Autodesk Inventor part; units mm, degrees
ref_plane "to_screw1_XY" through (15, 4.2426, 4.2426) normal (0, 0.7071, 0.7071) x (1, 0, 0)
ref_plane "to_screw1_YZ" through (15, 4.2426, 4.2426) normal (1, 0, 0) x (0, 0.7071, -0.7071)
ref_plane "to_screw1_ZX" through (15, 4.2426, 4.2426) normal (0, 0.7071, -0.7071) x (0, 0.7071, 0.7071)
sketch "Sketch_1" plane through (0, 0, 0) normal (0, 0, 1) x (1, 0, 0)
  line L0 (24, 0) -> (0, 0)
  line L1 (0, 18) -> (0, 6)
  line L2 (0, 6) -> (24, 6)
  line L3 (24, 6) -> (24, 8)
  line L4 (24, 8) -> (6, 8)
  line L5 (6, 8) -> (6, 18)
  line L6 (6, 18) -> (0, 18)
revolve "Revolution1" add sketch "Sketch_1" angle 360 about axis through (24, 0, 0) along (1, 0, 0)
sketch "Sketch_3" plane through (0, 0, 0) normal (0, -0.7071, 0.7071) x (1, 0, 0)
  line L0 (15, 5.5) -> (15, 8)
  line L1 (15, 8) -> (17, 8)
  line L2 (17, 8) -> (16.621, 7.621)
  line L3 (16.621, 7.621) -> (16.621, 5.5)
  line L4 (16.621, 5.5) -> (15, 5.5)
  line L5 (15, 5.5) -> (15, 8)
revolve "Revolution2" cut sketch "Sketch_3" angle 360 about axis through (15, 3.8891, 3.8891) along (0, -0.7071, -0.7071)
thread "Thread1"
sketch "Sketch_2" plane through (0, 0, 0) normal (0, -0.7071, -0.7071) x (1, 0, 0)
  line L0 (15, 5.5) -> (15, 8)
  line L1 (15, 8) -> (17, 8)
  line L2 (17, 8) -> (16.621, 7.621)
  line L3 (16.621, 7.621) -> (16.621, 5.5)
  line L4 (16.621, 5.5) -> (15, 5.5)
  line L5 (15, 5.5) -> (15, 8)
revolve "Revolution3" cut sketch "Sketch_2" angle 360 about axis through (15, -3.8891, 3.8891) along (0, 0.7071, -0.7071)
thread "Thread2"
sketch "Sketch_4" plane through (0, 0, 0) normal (0, 0, 1) x (1, 0, 0)
  line L0 (6, 13) -> (0, 13)
  line L1 (0, 13) -> (0, 15)
  line L2 (0, 15) -> (0.379, 14.621)
  line L3 (0.379, 14.621) -> (5.621, 14.621)
  line L4 (5.621, 14.621) -> (6, 15)
  line L5 (6, 15) -> (6, 13)
  line L6 (6, 13) -> (0, 13)
revolve "Revolution4" cut sketch "Sketch_4" angle 360 about axis through (6, 13, 0) along (1, 0, 0)
thread "Thread3"
sketch "Sketch_9" plane through (0, 0, 0) normal (0, -1, 0) x (1, 0, 0)
  line L0 (0, -13) -> (6, -13)
  line L1 (6, -13) -> (6, -15)
  line L2 (6, -15) -> (5.621, -14.621)
  line L3 (5.621, -14.621) -> (0.379, -14.621)
  line L4 (0.379, -14.621) -> (0, -15)
  line L5 (0, -15) -> (0, -13)
  line L6 (0, -13) -> (6, -13)
revolve "Revolution5" cut sketch "Sketch_9" angle 360 about axis through (0, 0, -13) along (-1, 0, 0)
thread "Thread4"
sketch "Sketch_10" plane through (0, 0, 0) normal (0, 0, 1) x (1, 0, 0)
  line L0 (0, -13) -> (6, -13)
  line L1 (6, -13) -> (6, -15)
  line L2 (6, -15) -> (5.621, -14.621)
  line L3 (5.621, -14.621) -> (0.379, -14.621)
  line L4 (0.379, -14.621) -> (0, -15)
  line L5 (0, -15) -> (0, -13)
  line L6 (0, -13) -> (6, -13)
revolve "Revolution6" cut sketch "Sketch_10" angle 360 about axis through (0, -13, 0) along (-1, 0, 0)
thread "Thread5"
sketch "Sketch_11" plane through (0, 0, 0) normal (0, -1, 0) x (1, 0, 0)
  line L0 (6, 13) -> (0, 13)
  line L1 (0, 13) -> (0, 15)
  line L2 (0, 15) -> (0.379, 14.621)
  line L3 (0.379, 14.621) -> (5.621, 14.621)
  line L4 (5.621, 14.621) -> (6, 15)
  line L5 (6, 15) -> (6, 13)
  line L6 (6, 13) -> (0, 13)
revolve "Revolution7" cut sketch "Sketch_11" angle 360 about axis through (6, 0, 13) along (1, 0, 0)
thread "Thread6"
ref_plane "to_screw1_XY" through (15, 4.2426, 4.2426) normal (0, 0.7071, 0.7071) x (1, 0, 0)
ref_plane "to_screw1_YZ" through (15, 4.2426, 4.2426) normal (1, 0, 0) x (0, 0.7071, -0.7071)
ref_plane "to_screw1_ZX" through (15, 4.2426, 4.2426) normal (0, 0.7071, -0.7071) x (0, 0.7071, 0.7071)
ref_plane "to_screw2_XY" through (15, -4.2426, 4.2426) normal (0, -0.7071, 0.7071) x (1, 0, 0)
ref_plane "to_screw2_YZ" through (15, -4.2426, 4.2426) normal (1, 0, 0) x (0, 0.7071, 0.7071)
ref_plane "to_screw2_ZX" through (15, -4.2426, 4.2426) normal (0, 0.7071, 0.7071) x (0, -0.7071, 0.7071)
properties part number "SSTHRT12-MB_b"
Source: CAD feature listing. Evaluate the final solid. Frame: model axes, mm. A direction names the side the tool comes from. Coordinates: 2 decimals unless noted, no trailing zeros. Loops run counter-clockwise (first coordinate to the right, second up) from the corner with the lowest first, then second, coordinate; pieces in that order, holes last. Notation, with made-up numbers: (15, 54) - (19, 54) arc R5 cw to (19, 61) - close; hole circle Ø10 at (8.25, 80.25). An arc over 180 degrees is marked (long way). Answer as CSV lines item,"result".
1. Section B-B (z = 13). Return loops of the section in (x, y), then the cut area to 3 significant figures.
Established:
outline,"(0, -12.45) - (6, -12.45) - (6, -2) - (5.62, -1.62) - (0.38, -1.62) - (0, -2) - close; (0, 2) - (0.38, 1.62) - (5.62, 1.62) - (6, 2) - (6, 12.45) - (0, 12.45) - close"
area,"130 mm2"
2. Contact query for flat-ended pins moving along their axis: pin 1 (5 mm diameter, centred on x = 15, z = -7.5, fed in from -Y) (3 decimals); pin 2 (6 mm diameter, centred on x = 7, z = -5.5, fed in from -Y); pin 3 (10 mm diameter, centred on x = 5, y = -9.5, fed in from +Z). Output: stop coordinate, or through.
Established:
pin 1,"stops at y = -6.245"
pin 2,"stops at y = -17.8"
pin 3,"stops at z = 17.43"
3. Section C-C (x = 21.25). Return loops of the section in (y, z).
Established:
outline,"circle Ø16 at (0, 0); hole circle Ø12 at (0, 0)"
4. Section A-A (y = 0). Return loops of the section in (x, z), then the cut area to 3 significant figures.
Established:
outline,"(0, -18) - (6, -18) - (6, -15) - (5.62, -14.62) - (0.38, -14.62) - (0, -15) - close; (0, -11) - (0.38, -11.38) - (5.62, -11.38) - (6, -11) - (6, -8) - (24, -8) - (24, -6) - (0, -6) - close; (0, 6) - (24, 6) - (24, 8) - (6, 8) - (6, 11) - (5.62, 11.38) - (0.38, 11.38) - (0, 11) - close; (0, 15) - (0.38, 14.62) - (5.62, 14.62) - (6, 15) - (6, 18) - (0, 18) - close"
area,"177 mm2"
5. Mould query, pull axis X, two halves, no side actions, for faces 3 (the flat face through (24, -2, 6)), 4 (the cylindrical face through (2.958, -2.343, -17.847)), 5 (the cylindrical face through (16.546, 4.383, 5.072)). Classes: released by +X, released by -X, zero draft, split by the parting line, or undercut.
Established:
face 3,"released by +X"
face 4,"zero draft"
face 5,"undercut"
6. Reachability of faces 1 (the cylindrical face through (14.87, 7.63, -2.4)), 2 (the cylindrical face through (16.546, -5.072, 4.383)) from +Z, -Z, +X, -X, +Y, -Y: full face, straight path, thin tool, end or side. Return the list, or none.
Established:
face 1,"+X"
face 2,"none"
7. Ray query, line 1 (Z direction, x = 2.1, y = 0); line 2 (Z direction, x = 4.25, y = -0.5); line 3 (Z direction, x = 14.25, y = -3.5). Return the intervals inside material, ascending.
Established:
line 1,"z = -18 to -14.62, -11.38 to -6, 6 to 11.38, 14.62 to 18"
line 2,"z = -17.99 to -14.54, -11.46 to -5.98, 5.98 to 11.46, 14.54 to 17.99"
line 3,"z = -7.19 to -4.87, 5.53 to 7.19"
